Read the model definition and answer for the solid it produces. Units are mm, in the model's axes. A direction names the side the tool comes from. Coordinates: 2 decimals unless noted, no trailing zeros. Loops run counter-clockwise (first coordinate to the right, second up) from the corner with the lowest first, then second, coordinate; pieces in that order, holes last.
from build123d import *

# Parameters (mm, degrees)
BOSS_EXTRU_2_DEPTH = 5


with BuildPart() as part:
    # Esquisse3D1 → Boss.-Extru.2 (new body)
    with BuildSketch(Plane(origin=(0, 0, -20), x_dir=(0.440651848036545, -0.8252970730775361, 0.35314400744119906), z_dir=(0, -0.39339715689728005, -0.9193686295198118))):
        Polygon((0, 0), (2.064889772, 9.784489268), (-2.827354862, 10.816934154), (-0.76246509, 20.601423421), (4.129779544, 19.568978535), (11.865292841, 56.223742318), (6.973048207, 57.256187204), (9.037937979, 67.040676471), (13.930182613, 66.008231585), (17.027517271, 80.684965487), (26.812006539, 78.620075715), (30.528808128, 96.232156396), (74.821304729, 96.775888054), (122.326612599, 0), (94.804862198, -34.708416185), (78.59808061, -26.876415767), (74.246969266, -35.880183316), (60.741317943, -29.353516301), (58.565762271, -33.855400075), (49.561994722, -29.504288732), (51.737550394, -25.002404957), (18.007535098, -8.702222687), (15.831979426, -13.204106461), (6.828211877, -8.852995118), (9.003767549, -4.351111343), align=None)
    extrude(amount=BOSS_EXTRU_2_DEPTH)


solid = part.part
Item 1: Find the intervals of material crossed by line 1 along Z through (x, y) = (6.5, -30); line 2 along Z through (x, y) = (38, -76); line 3 along X through (y, z) = (-8.5, -17.5), in increasing order.
Numbers:
line 1: z = -12.6 to -7.16
line 2: z = 7.08 to 12.52
line 3: x = -18.51 to 18.51
Item 2: A cutting plane is placed at A-A on x = -60.5. Determine the outline of the cut face in (y, z).
Numbers:
outline: (-90.17, 13.15) - (-57.2, -0.96) - (-55.23, 3.63) - (-88.21, 17.74) - close; (-53.9, -2.37) - (-45.52, -5.96) - (-43.55, -1.36) - (-51.94, 2.22) - close
Item 3: A cutting plane is placed at C-C on x = -31.5. Determine the outline of the cut face in (y, z).
Numbers:
outline: (-102.92, 18.6) - (-24.64, -14.89) - (-22.68, -10.3) - (-100.96, 23.2) - close
Item 4: A cutting plane is placed at B-B on y = -25. Determine the outline of the cut face in (x, z), then the cut area to 3 significant figures.
Numbers:
outline: (-34.73, -9.3) - (-31.99, -14.74) - (31.99, -14.74) - (34.73, -9.3) - close
area: 363 mm2
Item 5: Determine the mould class of faces 1 (the face through (17.27, -10.52, -18.18)), 2 (the face through (-54.68, -37.37, -6.69)), 3 (the face through (46.805, -31.705, -9.115)) for opening direction X: released by +X, released by -X, zero draft, split by the parting line, or undercut.
Numbers:
face 1: released by +X
face 2: released by -X
face 3: undercut
Item 6: Given pin 1 (5 mm diameter, centred on x = 40, z = 10.5, fed in from +Y); pin 2 (6 mm diameter, centred on x = 33.5, z = -10, fed in from -Y); pin 3 (1 mm diameter, centred on x = -16.5, z = 7.5, fed in from +Y), each flat-ended and moving along its own axis, determine where each tip first touches the part or whether it passes through.
Numbers:
pin 1: stops at y = -65.44
pin 2: stops at y = -43.09
pin 3: stops at y = -63.1
Item 7: Which of the six approach directions +Z, -Z, +X, -X, +Y, -Y give full straight-line access (tool end or side, diameter ignored) to faces 4 (the face through (-17.31, -10.47, -18.2)), 5 (the face through (54.64, -37.42, -6.67)), 6 (the face through (-1.45, -62.75, 6.85)), 7 (the face through (-3.88, -3.76, -21.07))?
Numbers:
face 4: -X
face 5: +X
face 6: +Z, +X, -X, +Y
face 7: -Z, +Y
